Could you check a few things on this model? Use its own coordinates, in mm. Face numbers are marked on the shaded views. A direction names the side the tool comes from. Give positions to 0.01 mm unless a question says otherwise; leave off trailing zeros. Order: outer loops, then holes, each group sorted by start corner. A loop starts at its lowest first (then second) coordinate and runs counter-clockwise, first axis right, second up.
(1) Imagine slicing it at B-B, the plane y = 29. Write out the boundary of the cut face in (x, z), then the cut area to 3 significant figures.
(2) Imagine slicing it at D-D, the plane y = -5.5. Write out the boundary of the cut face in (x, z) (3 decimals), then the cut area to 3 significant figures.
(3) If we mould it in two halves opening along Z, with no side actions, what happens to the marked faces 6, 7 and 8? For each: released by +Z, released by -Z, zero draft, split by the parting line, or undercut.
(4) Imagine slicing it at A-A, the plane x = 0. Write out the boundary of the cut face in (y, z) (3 decimals), then the cut area to 3 significant figures.
(5) If I drill on probe 1 along Z at (x, y) = (2.5, 33); probe 2 along Y at (x, z) = (9, -10.5); probe 3 along Y at (x, z) = (10.5, 5.5), over which ranges is the centre line in solid material (lowest first)?
(6) Imagine slicing it at C-C, the plane z = 0. Write out the boundary of the cut face in (x, y) (3 decimals).
(7) On a 3-axis mill with a long thin cutter (end or side, diameter ignored), from which of +Z, -Z, +X, -X, +Y, -Y can I reach the whole of each face in a straight line? I mean the marked faces 1, 2, 3, 4 and 5. Say none if no direction works.
(8) Will these pins go through, and if not, where does the flat tip stop? pin 1 (7.5 mm diameter, centred on y = 40, z = 1.5, fed in from +X); pin 2 (5 mm diameter, centred on x = 1, y = 49, fed in from -Z); pin 3 (8 mm diameter, centred on x = 1, y = 50.5, fed in from +Z); pin 4 (12 mm diameter, centred on x = 9, z = -12, fed in from +Y).
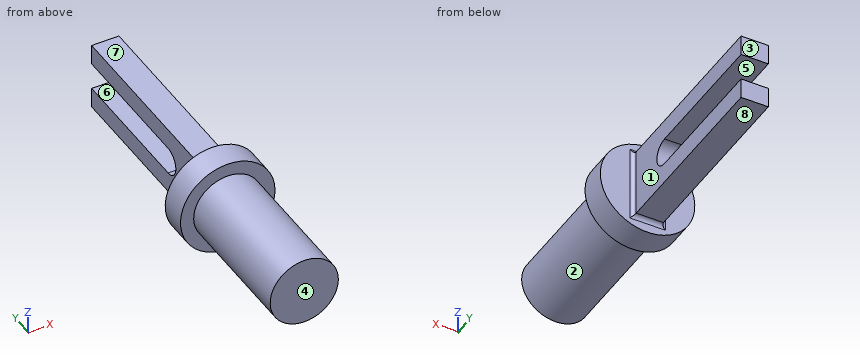
from build123d import *

# Parameters (mm, degrees)
SKETCH1_R           = 17.325
BOSS_EXTRUDE1_DEPTH = 10
SKETCH2_R           = 12.5
BOSS_EXTRUDE2_DEPTH = 50
SKETCH3_W           = 10
SKETCH3_H           = 25
BOSS_EXTRUDE3_DEPTH = 70
FILLET1_R           = 1.5
CUT_EXTRUDE1_DEPTH  = 76.488815397


with BuildPart() as part:
    # Sketch1 → Boss-Extrude1 (new body)
    with BuildSketch(Plane(origin=(0, 0, 0), x_dir=(1, 0, 0), z_dir=(0, 1, 0))):
        with Locations(Location((0, 0, 0), (0, 0, 270))):
            Circle(SKETCH1_R)
    extrude(amount=-BOSS_EXTRUDE1_DEPTH)

    # Sketch2 → Boss-Extrude2 (add)
    with BuildSketch(Plane.XZ.offset(10)):
        with Locations(Location((0, 0, 0), (0, 0, 270))):
            Circle(SKETCH2_R)
    extrude(amount=BOSS_EXTRUDE2_DEPTH)

    # Sketch3 → Boss-Extrude3 (add)
    with BuildSketch(Plane(origin=(0, 0, 0), x_dir=(1, 0, 0), z_dir=(0, 1, 0))):
        Rectangle(SKETCH3_W, SKETCH3_H)
    extrude(amount=BOSS_EXTRUDE3_DEPTH)

    # Fillet1
    fillet1_edges = [part.edges().sort_by_distance(p)[0] for p in [
        (5, 0, 0),
        (0, 0, -12.5),
        (-5, 0, 0),
        (0, 0, 12.5),
    ]]
    fillet(fillet1_edges, radius=FILLET1_R)

    # Sketch4 → Cut-Extrude1 (cut, through all)
    with BuildSketch(Plane.ZY.offset(5)):
        with BuildLine():
            Line((5, 70), (-5, 70))
            Line((-5, 70), (-5, 20))
            ThreePointArc((-5, 20), (0, 15), (5, 20))
            Line((5, 20), (5, 70))
        make_face()
    extrude(amount=-CUT_EXTRUDE1_DEPTH, mode=Mode.SUBTRACT)


solid = part.part
Answer block:
1. outline: (-5, -12.5) - (5, -12.5) - (5, -5) - (-5, -5) - close; (-5, 5) - (5, 5) - (5, 12.5) - (-5, 12.5) - close
1. area: 150 mm2
2. outline: circle Ø34.65 at (0, 0)
2. area: 943 mm2
3. face 6: undercut
3. face 7: released by +Z
3. face 8: released by -Z
4. outline: (-60, -12.5) - (-10, -12.5) - (-10, -17.325) - (0, -17.325) - (0, -14) arc R1.5 cw to (1.5, -12.5) - (70, -12.5) - (70, -5) - (20, -5) arc R5 cw to (20, 5) - (70, 5) - (70, 12.5) - (1.5, 12.5) arc R1.5 cw to (0, 14) - (0, 17.325) - (-10, 17.325) - (-10, 12.5) - (-60, 12.5) - close
4. area: 2,810 mm2
5. probe 1: z = -12.5 to -5, 5 to 12.5
5. probe 2: y = -10 to 0
5. probe 3: y = -60 to 0
6. outline: (-17.325, -10) - (-12.5, -10) - (-12.5, -60) - (12.5, -60) - (12.5, -10) - (17.325, -10) - (17.325, 0) - (6.5, 0) arc R1.5 cw to (5, 1.5) - (5, 15) - (-5, 15) - (-5, 1.5) arc R1.5 cw to (-6.5, 0) - (-17.325, 0) - close
7. face 1: +Z, -Z, +X, +Y
7. face 2: -Y
7. face 3: +Z, -Z, +X, -X, +Y
7. face 4: +Z, -Z, +X, -X, -Y
7. face 5: +X, -X, +Y
8. pin 1: stops at x = 5
8. pin 2: stops at z = -12.5
8. pin 3: stops at z = 12.5
8. pin 4: stops at y = 70
